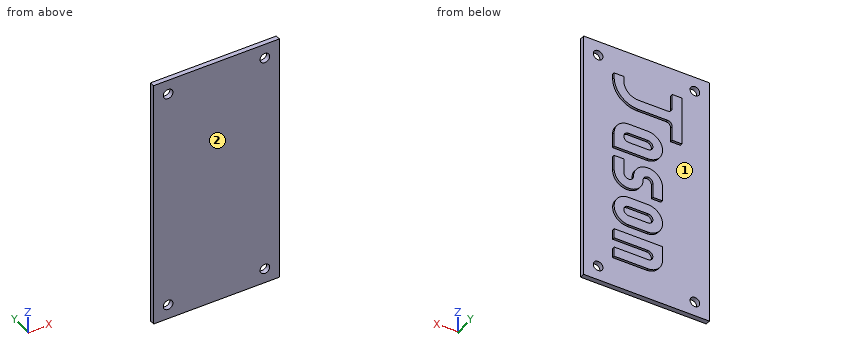
Autodesk Inventor part; units mm, degrees
ref_plane "YZ Plane" through (0, 0, 0) normal (1, 0, 0) x (0, 1, 0)
ref_plane "XZ Plane" through (0, 0, 0) normal (0, 1, 0) x (-1, 0, 0)
ref_plane "XY Plane" through (0, 0, 0) normal (0, 0, 1) x (1, 0, 0)
sketch "Sketch1" plane through (0, 0, 0) normal (0, 1, 0) x (-1, 0, 0)
  line L0 (-82.55, -165.1) -> (0, -165.1)
  line L1 (0, -165.1) -> (0, 0)
  line L2 (0, 0) -> (-82.55, 0)
  line L3 (-82.55, 0) -> (-82.55, -165.1)
  circle A0 centre (-73.025, -155.575) radius 3.175
  circle A1 centre (-73.025, -155.575) radius 3.175
  circle A2 centre (-9.525, -155.575) radius 3.175
  circle A3 centre (-9.525, -155.575) radius 3.175
  circle A4 centre (-73.025, -9.525) radius 3.175
  circle A5 centre (-73.025, -9.525) radius 3.175
  circle A6 centre (-9.525, -9.525) radius 3.175
  circle A7 centre (-9.525, -9.525) radius 3.175
extrude "Extrusion1" add sketch "Sketch1" along normal blind 3.175
sketch "Sketch2" plane through (0, 3.175, 0) normal (0, 1, 0) x (1, 0, 0)
  line L0 (63.5, 19.05) -> (57.15, 19.05)
  line L1 (57.15, 19.05) -> (57.15, 22.225)
  line L2 (63.5, 19.05) -> (63.5, 22.225)
  arc A0 (57.15, 22.225) -> (47.625, 31.75) centre (47.625, 22.225) ccw
  arc A1 (63.5, 22.225) -> (47.625, 38.1) centre (47.625, 22.225) ccw
  line L3 (47.625, 31.75) -> (28.575, 31.75)
  line L4 (28.575, 38.1) -> (47.625, 38.1)
  arc A2 (28.575, 31.75) -> (25.4, 28.575) centre (28.575, 28.575) ccw
  arc A3 (25.4, 41.275) -> (28.575, 38.1) centre (28.575, 41.275) ccw
  line L5 (25.4, 19.05) -> (25.4, 28.575)
  line L6 (25.4, 19.05) -> (19.05, 19.05)
  line L7 (25.4, 41.275) -> (25.4, 50.8)
  line L8 (25.4, 50.8) -> (19.05, 50.8)
  line L9 (19.05, 50.8) -> (19.05, 19.05)
  point P0 (0, 0)
sketch "Sketch3" plane through (0, 3.175, 0) normal (0, 1, 0) x (1, 0, 0)
  point P0 (0, 0)
extrude "Extrusion2" add sketch "Sketch2" along normal blind 1.5875
sketch "Sketch4" plane through (0, 3.175, 0) normal (0, 1, 0) x (1, 0, 0)
  arc A0 (53.975, 57.15) -> (53.975, 63.5) centre (53.975, 60.325) ccw
  line L0 (53.975, 57.15) -> (41.275, 57.15)
  arc A1 (41.275, 63.5) -> (41.275, 57.15) centre (41.275, 60.325) ccw
  line L1 (41.275, 63.5) -> (53.975, 63.5)
  arc A2 (53.975, 50.8) -> (63.5, 60.325) centre (53.975, 60.325) ccw
  line L2 (53.975, 50.8) -> (41.275, 50.8)
  arc A3 (41.275, 69.85) -> (41.275, 50.8) centre (41.275, 60.325) ccw
  line L3 (41.275, 69.85) -> (63.5, 69.85)
  line L4 (63.5, 69.85) -> (63.5, 60.325)
  line L5 (57.15, 76.2) -> (63.5, 76.2)
  line L6 (63.5, 76.2) -> (63.5, 85.725)
  line L7 (57.15, 76.2) -> (57.15, 85.725)
  arc A4 (57.15, 85.725) -> (50.8, 85.725) centre (53.975, 85.725) ccw
  arc A5 (63.5, 85.725) -> (44.45, 85.725) centre (53.975, 85.725) ccw
  arc A6 (38.1, 85.725) -> (44.45, 85.725) centre (41.275, 85.725) ccw
  line L8 (31.75, 95.25) -> (38.1, 95.25)
  line L9 (38.1, 95.25) -> (38.1, 85.725)
  line L10 (41.275, 107.95) -> (53.975, 107.95)
  arc A7 (41.275, 114.3) -> (41.275, 107.95) centre (41.275, 111.125) ccw
  arc A8 (53.975, 107.95) -> (53.975, 114.3) centre (53.975, 111.125) ccw
  line L11 (53.975, 114.3) -> (41.275, 114.3)
  arc A9 (41.275, 120.65) -> (41.275, 101.6) centre (41.275, 111.125) ccw
  line L12 (41.275, 101.6) -> (53.975, 101.6)
  arc A10 (53.975, 101.6) -> (53.975, 120.65) centre (53.975, 111.125) ccw
  line L13 (53.975, 120.65) -> (41.275, 120.65)
  line L14 (63.5, 127) -> (63.5, 133.35)
  line L15 (63.5, 133.35) -> (41.275, 133.35)
  arc A11 (41.275, 139.7) -> (41.275, 133.35) centre (41.275, 136.525) ccw
  line L16 (41.275, 139.7) -> (63.5, 139.7)
  line L17 (63.5, 139.7) -> (63.5, 146.05)
  line L18 (63.5, 146.05) -> (41.275, 146.05)
  arc A12 (41.275, 146.05) -> (31.75, 136.525) centre (41.275, 136.525) ccw
  line L19 (63.5, 127) -> (31.75, 127)
  line L20 (31.75, 127) -> (31.75, 136.525)
  line L21 (57.15, 19.05) -> (57.15, 22.225)
  arc A13 (57.15, 22.225) -> (47.625, 31.75) centre (47.625, 22.225) ccw
  line L22 (47.625, 31.75) -> (28.575, 31.75)
  arc A14 (28.575, 31.75) -> (25.4, 28.575) centre (28.575, 28.575) ccw
  line L23 (25.4, 28.575) -> (25.4, 19.05)
  line L24 (25.4, 19.05) -> (19.05, 19.05)
  line L25 (19.05, 19.05) -> (19.05, 50.8)
  line L26 (19.05, 50.8) -> (25.4, 50.8)
  line L27 (25.4, 50.8) -> (25.4, 41.275)
  arc A15 (25.4, 41.275) -> (28.575, 38.1) centre (28.575, 41.275) ccw
  line L28 (28.575, 38.1) -> (47.625, 38.1)
  arc A16 (63.5, 22.225) -> (47.625, 38.1) centre (47.625, 22.225) ccw
  line L29 (63.5, 22.225) -> (63.5, 19.05)
  line L30 (63.5, 19.05) -> (57.15, 19.05)
  circle A17 centre (9.525, 9.525) radius 3.175
  circle A18 centre (73.025, 9.525) radius 3.175
  circle A19 centre (9.525, 155.575) radius 3.175
  circle A20 centre (73.025, 155.575) radius 3.175
  line L31 (82.55, 165.1) -> (0, 165.1)
  line L32 (0, 165.1) -> (0, 0)
  line L33 (0, 0) -> (82.55, 0)
  line L34 (82.55, 0) -> (82.55, 165.1)
  line L35 (31.75, 95.25) -> (31.75, 85.725)
  arc A21 (31.75, 85.725) -> (50.8, 85.725) centre (41.275, 85.725) ccw
extrude "Extrusion3" add sketch "Sketch4" along normal blind 1.5875 contours L2 A3 L3 L4 A2 | L7 A4 A21 L35 L8 L9 A6 A5 L6 L5 | L13 A10 L12 A9 | L19 L20 A12 L18 L17 L16 A11 L15 L14
properties part number "JASON"
Geometry: final body of the model. Coordinates: model frame, mm. Face numbers are marked on the shaded views. Give positions to 0.01 mm unless a question says otherwise; leave off trailing zeros. Loops run counter-clockwise (first coordinate to the right, second up) from the corner with the lowest first, then second, coordinate; pieces in that order, holes last. Notation, with made-up numbers: (26.25, -32.5) -> (62.25, -32.5) arc R14 cw to (62.25, -27.5) -> close; hole circle Ø6 at (-4, -11). An arc over 180 degrees is marked (long way). Put each result on its own line as item: value.
1. Cut plane C-C (z = -122.5). Return the cut outline in (x, y) (3 decimals).
Taken from the geometry:
outline: (0, 0) -> (82.55, 0) -> (82.55, 3.175) -> (0, 3.175) -> close
2. Pull-direction query (Z, two-part tool) for the marked faces 1 and 2; classes: released by +Z, released by -Z, zero draft, split by the parting line, or undercut.
Taken from the geometry:
face 1: undercut
face 2: zero draft
3. Cut plane B-B (x = 65.5). Return the cut outline in (y, z) (3 decimals).
Taken from the geometry:
outline: (0, -165.1) -> (3.175, -165.1) -> (3.175, 0) -> (0, 0) -> close
4. Ray query, line 1 along Z through (x, y) = (72.5, 2.15); line 2 along Y through (x, z) = (16.5, -146) (3 decimals); line 3 along X through (y, z) = (4.2, -142.5). Return the intervals inside material, ascending. Write a range as [from, to].
Taken from the geometry:
line 1: z = [-165.1, -158.71], [-152.44, -12.66], [-6.39, 0]
line 2: y = [0, 3.175]
line 3: x = [33.86, 63.5]
5. Pin query (flat end, axial travel): P1, Ø1.3, axis at x = 39.5, y = 3.5, coming from the +Z side; P2, Ø1.7, axis at x = 40, y = 4.5, coming from the -Z side; P3, Ø8, axis at x = 72, z = -140.5, coming from the +Y side (3 decimals); P4, Ø1.3, axis at x = 48.5, y = 4, coming from the +Z side. Return the tip coordinate at first contact, or that it passes through.
Taken from the geometry:
P1: stops at z = 0
P2: stops at z = -146.04
P3: stops at y = 3.175
P4: stops at z = -31.63
